Source: CAD feature listing. Evaluate the final solid. Frame: model axes, mm. A direction names the side the tool comes from. Round coordinates to 2 decimals unless told otherwise and drop trailing zeros. Order: outer loops, then holes, each group sorted by start corner. A loop starts at its lowest first (then second) coordinate and runs counter-clockwise, first axis right, second up. Notation, with made-up numbers: (85.25, 71.25) - (119.25, 71.25) arc R25 ccw to (119.25, 104.25) - close; hole circle Ø1 at (46, 36). An arc over 180 degrees is marked (long way). Use one line per item in the form item = value. Start each with the question number.
Q1. Draft query along Z for faces 5 (the flat face through (-28, -20, 28)), 6 (the flat face through (-81, -59, 40)), 7 (the flat face through (2, -1, -120)), 8 (the flat face through (41, 20, -34)). Return one class per face: released by +Z, released by -Z, zero draft, split by the parting line, or undercut.
Q2. Cut plane A-A, the plane x = -59. Return the cut outline in (y, z).
Q3. Cut plane B-B, the plane y = 27.5. Return the cut outline in (x, z), and give its area (3 significant figures).
Q4. Cut plane D-D, the plane x = -10.5. Return the cut outline in (y, z), and give its area (3 significant figures).
Q5. Pin query (flat end, axial travel): pin 1 Ø20 at (x, y) = (96.5, 15) entering from +Z; pin 2 Ø10 at (x, z) = (5.5, 74) entering from +Y; pin 3 Ø20 at (x, z) = (81, 63.5) entering from +Y. Return the tip coordinate at first contact, or that it passes through.
Q6. Set-up query: faces 1 (the flat face through (-40, -59, 79)), 2 (the flat face through (88, 60, 60)), 3 (the flat face through (-21, 12, -21)), 4 (the flat face through (81, 40, 40)). Return all of +Z, -Z, +X, -X, +Y, -Y with unobstructed straight access to the full face (end or side cutting, diameter ignored); none if empty.
Q7. Ray query, line 1 (Z direction, x = -89, y = -48.5); line 2 (Z direction, x = 25.5, y = 74); line 3 (X direction, y = -84.5, z = 74.5). Return the intervals inside material, ascending. Write a range as [from, to].
Q8. Cut plane C-C, the plane z = -46. Return the cut outline in (x, y).
from build123d import *

# Parameters (mm, degrees)
BOSS_EXTRUDE1_DEPTH = 120
SKETCH1_3_W         = 80
SKETCH1_3_H         = 80
BOSS_EXTRUDE2_DEPTH = 40
BOSS_EXTRUDE3_DEPTH = 120
SKETCH1_5_W         = 80
SKETCH1_5_H         = 80
BOSS_EXTRUDE4_DEPTH = 120
BOSS_EXTRUDE7_DEPTH = 80
BOSS_EXTRUDE8_DEPTH = 120
BOSS_EXTRUDE9_DEPTH = 40


with BuildPart() as part:
    # Sketch1 → Boss-Extrude1 (new body)
    with BuildSketch(Plane.XY):
        Polygon((120, -100), (120, -20), (80, -20), (-40, -20), (-40, -100), align=None)
    extrude(amount=BOSS_EXTRUDE1_DEPTH)

    # Sketch1<3> → Boss-Extrude2 (add)
    with BuildSketch(Plane.XY):
        with Locations((-80, -60)):
            Rectangle(SKETCH1_3_W, SKETCH1_3_H)
    extrude(amount=BOSS_EXTRUDE2_DEPTH)

    # Sketch1<4> → Boss-Extrude3 (add)
    with BuildSketch(Plane.XY):
        Polygon((120, -100), (120, -20), (80, -20), (-40, -20), (-40, -100), align=None)
    extrude(amount=-BOSS_EXTRUDE3_DEPTH)

    # Sketch1<5> → Boss-Extrude4 (add)
    with BuildSketch(Plane.XY):
        with Locations((-80, -60)):
            Rectangle(SKETCH1_5_W, SKETCH1_5_H)
    extrude(amount=-BOSS_EXTRUDE4_DEPTH)

    # Sketch4 → Boss-Extrude7 (add)
    with BuildSketch(Plane(origin=(0, -20, 0), x_dir=(1, 0, 0), z_dir=(0, 1, 0))):
        Polygon((80, -80), (120, -80), (120, -40), (40, -40), align=None)
    extrude(amount=BOSS_EXTRUDE7_DEPTH)

    # Sketch4<3> → Boss-Extrude8 (add)
    with BuildSketch(Plane(origin=(0, -20, 0), x_dir=(1, 0, 0), z_dir=(0, 1, 0))):
        Polygon((-80, 80), (120, 80), (120, 120), (-120, 120), align=None)
    extrude(amount=BOSS_EXTRUDE8_DEPTH)

    # Sketch4<4> → Boss-Extrude9 (add)
    with BuildSketch(Plane(origin=(0, -20, 0), x_dir=(1, 0, 0), z_dir=(0, 1, 0))):
        Polygon((40, -40), (120, -40), (120, 80), (-80, 80), align=None)
    extrude(amount=BOSS_EXTRUDE9_DEPTH)


solid = part.part
Completed:
q1.face_5 = zero draft
q1.face_6 = released by +Z
q1.face_7 = released by -Z
q1.face_8 = undercut
q2.outline = (-100, -120) - (100, -120) - (100, -80) - (20, -80) - (20, -59) - (-20, -59) - (-20, 40) - (-100, 40) - close
q3.outline = (-120, -120) - (120, -120) - (120, -80) - (-80, -80) - close; (40, 40) - (120, 40) - (120, 80) - (80, 80) - close
q3.area = 11,200 mm2
q4.outline = (-100, -120) - (100, -120) - (100, -80) - (20, -80) - (20, -10.5) - (-20, -10.5) - (-20, 120) - (-100, 120) - close
q4.area = 26,800 mm2
q5.pin_1 = 80
q5.pin_2 = -20
q5.pin_3 = 60
q6.face_1 = +Z, -X, +Y, -Y
q6.face_2 = +Z, +X, -X, +Y
q6.face_3 = +Z, -X, +Y
q6.face_4 = +X, -X, +Y
q7.line_1 = [-120, 40]
q7.line_2 = [-120, -80]
q7.line_3 = [-40, 120]
q8.outline = (-120, -100) - (120, -100) - (120, 20) - (-46, 20) - (-46, -20) - (-120, -20) - close
